The model under review builds one solid part; all positions refer to its coordinate system, in mm. A direction names the side the tool comes from. Round coordinates to 2 decimals unless told otherwise and drop trailing zeros. Order: outer loops, then holes, each group sorted by start corner. A loop starts at its lowest first (then second) coordinate and runs counter-clockwise, first axis right, second up.
1) Mouldability with a two-part tool opening along X and no side actions: class faces 1 (the face through (1.014, 6.466, -2.681)), 2 (the face through (2, -6, 4)), 3 (the face through (11.27, -6.597, -2.733)), 4 (the face through (8.5, 7, 0)) as pulls with the +X half, pulls with the -X half, needs draft (parallel to the pull), parting line crosses it, or undercut.
2) Consider section D-D (z = -3.5). Give the boundary of the cut face in (x, y).
3) Consider section B-B (y = 0). Give the boundary of the cut face in (x, z).
4) Consider section A-A (z = 0). Give the boundary of the cut face in (x, y), then the cut area to 3 significant figures.
5) Clearance check with flat-ended pins moving along their axes: P1, Ø3, axis at x = 11, z = -3.5, coming from the -Y side; P2, Ø2, axis at y = -3.5, z = -0.5, coming from the +X side; P3, Ø1.3, axis at x = 9.5, z = 5.5, coming from the +Y side; P4, Ø2, axis at x = 2.5, z = -6, coming from the +Y side. State where each tip first meets the part, or that it passes through.
6) Consider section C-C (y = 6). Give the boundary of the cut face in (x, z).
7) Machinability: for faces 5 (the face through (20, -3, 6)), 6 (the face through (10, 4.3, -6)), 7 (the face through (13.4, -7.16, 0.03)), 8 (the face through (9, -7, 0)), which of the approach directions +Z, -Z, +X, -X, +Y, -Y give a long, thin tool a straight path to every point of the face, cutting with its end or side? Answer none if there is none.
8) To check wall thickness, follow L1, parallel to Z at x = 13, y = 0; L2, parallel to Z at x = 11, y = -4.75. State the ranges of each line that lie inside material, in increasing order.
Autodesk Inventor part; units mm, degrees
ref_plane "YZ-Ebene" through (0, 0, 0) normal (1, 0, 0) x (0, 1, 0)
ref_plane "XY-Ebene" through (0, 0, 0) normal (0, 0, 1) x (1, 0, 0)
sketch "Skizze1" plane through (0, 0, 0) normal (0, 0, 1) x (1, 0, 0)
  line L0 (-4, 0) -> (24, 0)
  line L1 (0, -1.56) -> (0, 9.36)
  line L2 (0, 7) -> (2, 7)
  line L3 (2, 7) -> (2, 7.8)
  line L4 (2, 7.8) -> (20, 7.8)
  line L5 (20, 7.8) -> (20, 6.5)
  line L6 (20, 6.5) -> (0, 6.5)
  line L7 (0, 7) -> (0, 6.5)
  point P0 (0, 0)
  dimension "d0" = 6.5
  dimension "d1" = 7.8
  dimension "d2" = 7
  dimension "d3" = 2
  dimension "d4" = 20
revolve "Umdrehung1" add sketch "Skizze1" angle 360 about axis through (-10, 0, 0) along (1, 0, 0)
ref_plane "Arbeitsebene1" through (11, 7.8, 0) normal (0, 1, 0) x (-1, 0, 0)
sketch "Skizze2" plane through (11, 7.8, 0) normal (0, 1, 0) x (-1, 0, 0)
  line L0 (9, 7.8) -> (9, -7.8)
  line L1 (-9, 7.8) -> (-9, -7.8)
  line L2 (9, -7.8) -> (-9, -7.8)
  line L3 (9, 7.8) -> (-9, 7.8)
  line L4 (2.5, 10) -> (2.5, -10)
  line L5 (2.5, -10) -> (-1, -10)
  line L6 (-1, -10) -> (-1, 10)
  line L7 (-1, 10) -> (2.5, 10)
  line L8 (11, 7) -> (11, -7)
  line L9 (15, 0) -> (-13, 0)
  point P0 (11, 0)
  dimension "d6" = 20
  dimension "d7" = 3.5
  dimension "d8" = 8.5
extrude "Extrusion1" cut sketch "Skizze2" against normal blind 3.5 contours L4 L9 L6 L3 | L3 L6 L7 L4 | L4 L2 L6 L9 | L4 L5 L6 L2
sketch "Skizze3" plane through (0, 0, 0) normal (0, 0, 1) x (1, 0, 0)
  point P0 (0, 0)
sketch "Skizze4" plane through (0, 0, 0) normal (1, 0, 0) x (0, 1, 0)
  point P0 (0, 0)
sketch "Skizze5" plane through (0, 0, 0) normal (0, 0, 1) x (1, 0, 0)
  point P0 (0, 0)
sketch "Skizze6" plane through (0, 0, 0) normal (0, 0, 1) x (1, 0, 0)
  point P0 (0, 0)
sketch "Skizze7" plane through (0, 0, 0) normal (0, 0, 1) x (1, 0, 0)
  line L0 (2, -7.8) -> (20, -7.8)
  line L1 (12.982, -10.982) -> (6.618, -4.618)
  line L2 (15.1033, -8.8607) -> (12.982, -10.982)
  line L3 (6.618, -4.618) -> (8.7393, -2.4967)
  line L4 (15.1033, -8.8607) -> (8.7393, -2.4967)
  line L5 (20, -6.5) -> (20, 6.5)
  line L6 (-4, 0) -> (24, 0)
  point P0 (0, 0)
  point P1 (9.8, -7.8)
  dimension "d12" = 9
  dimension "d13" = 3
  dimension "d14" = 10.2
  dimension "d19" = 9
  dimension "d20" = 3
  dimension "d21" = 45
revolve "Umdrehung2" cut sketch "Skizze7" angle 45 mid plane about axis through (-10, 0, 0) along (1, 0, 0)
fillet "Rundung1" radius 0.6 4 edges at (13.3926, -6.6057, -2.7362) (13.3926, -6.6057, 2.7362) (9.15, -6.6057, 2.7362) (9.15, -6.6057, -2.7362)
properties part number "Zylinderbuchse_ra8846s" material "Stahl, Guss"
Answer below:
1. face 1: needs draft
1. face 2: pulls with the -X half
1. face 3: undercut
1. face 4: undercut
2. outline: (0, -6.06) - (2, -6.06) - (2, -6.97) - (20, -6.97) - (20, -5.48) - (0, -5.48) - close; (0, 5.48) - (8.5, 5.48) - (8.5, 6.97) - (2, 6.97) - (2, 6.06) - (0, 6.06) - close; (12, 5.48) - (20, 5.48) - (20, 6.97) - (12, 6.97) - close
3. outline: (0, -7) - (2, -7) - (2, -7.8) - (20, -7.8) - (20, -6.5) - (0, -6.5) - close; (0, 6.5) - (20, 6.5) - (20, 7.8) - (2, 7.8) - (2, 7) - (0, 7) - close
4. outline: (0, -7) - (2, -7) - (2, -7.8) - (9.8, -7.8) - (8.5, -6.5) - (0, -6.5) - close; (0, 6.5) - (8.5, 6.5) - (8.5, 7.8) - (2, 7.8) - (2, 7) - (0, 7) - close; (12, 6.5) - (20, 6.5) - (20, 7.8) - (12, 7.8) - close; (12.74, -6.5) - (14.04, -7.8) - (20, -7.8) - (20, -6.5) - close
4. area: 38.7 mm2
5. P1: stops at y = -7.37
5. P2: passes through
5. P3: stops at y = 4.3
5. P4: stops at y = 5.99
6. outline: (0, -3.61) - (2, -3.61) - (2, -4.98) - (8.5, -4.98) - (8.5, -2.5) - (0, -2.5) - close; (0, 2.5) - (8.5, 2.5) - (8.5, 4.98) - (2, 4.98) - (2, 3.61) - (0, 3.61) - close; (12, -4.98) - (20, -4.98) - (20, -2.5) - (12, -2.5) - close; (12, 2.5) - (20, 2.5) - (20, 4.98) - (12, 4.98) - close
7. face 5: +Z, -Z, +X, +Y, -Y
7. face 6: +Z, -Z, +Y
7. face 7: -Y
7. face 8: +Y
8. L1: z = -7.8 to -6.5, 6.5 to 7.8
8. L2: z = -6.19 to -4.44, 4.44 to 6.19
